Verification items for the finished model (mm, model axes). Face numbers are marked on the shaded views. A direction names the side the tool comes from. Round coordinates to 2 decimals unless told otherwise and drop trailing zeros. Write each loop counter-clockwise with the first axis right and the second up, starting at its lowest first coordinate (ties: lowest second). Pieces come first, ordered by that corner, then holes. Notation, with made-up numbers: M -23.5,9.5 L 4.5,9.5 A11 ccw 4.5,19.5 Z; hole C -4.5,20.5 d7. An arc over 180 degrees is marked long. Answer in a Markdown table with one row per item. Add a question column.
1. Material ranges on probe 1 along Z at (x, y) = (0, 0.55); probe 2 along X at (y, z) = (0.6, 25.5); probe 3 along Y at (x, z) = (0, 26.3), recorded low to high.
2. Sectioned sample at B-B on y = 3.75. Record the cut outline in (x, z).
3. Draft check along Y on the marked faces 1, 2 and 3. Enter one of: pulls with the +Y half, pulls with the -Y half, needs draft (parallel to the pull), parting line crosses it, or undercut.
4. Sectioned sample at A-A on z = 5.5. Record the cut outline in (x, y), plus the area to 3 significant figures.
5. Go/stop test with flat-tipped pins: pin 1 Ø1.2 at (y, z) = (0, 13.5) entering from -X; pin 2 Ø0.5 at (y, z) = (0, 8) entering from +X; pin 3 Ø0.7 at (x, z) = (0, 26) entering from +Y. Record where each tip stops, or that it passes through.
6. Sectioned sample at D-D on z = 25.5. Record the cut outline in (x, y), plus the area to 3 significant figures.
7. Set-up check for the marked faces 4, 5 and 6: record each of +Z, -Z, +X, -X, +Y, -Y from which the full face is reachable in a straight line by a thin tool's end or side.
8. Sectioned sample at C-C on y = 0.5. Record the cut outline in (x, z).
```python
from build123d import *

# Parameters (mm, degrees)
SKETCH1_R                = 0.66
SKETCH1_R_2              = 0.4
BOSS_EXTRUDE1_DEPTH      = 4
BOSS_EXTRUDE1_DEPTH_BACK = 1
BOSS_EXTRUDE2_DEPTH      = 20
SKETCH8_R                = 0.4
BOSS_EXTRUDE3_DEPTH      = 3
BOSS_EXTRUDE3_DEPTH_BACK = 20
FILLET1_R                = 0.5
CUT_EXTRUDE4_START       = -4
CUT_EXTRUDE4_DEPTH       = 4
CUT_EXTRUDE5_START       = -10
CUT_EXTRUDE5_DEPTH       = 4
CUT_EXTRUDE6_START       = -16
CUT_EXTRUDE6_DEPTH       = 4
CUT_EXTRUDE7_DEPTH       = 0.2
CHAMFER1_SIZE            = 0.2
CUT_EXTRUDE9_START       = -22
CUT_EXTRUDE9_DEPTH       = 4
SKETCH17_R               = 0.59
CUT_EXTRUDE11_DEPTH      = 9.61358644


with BuildPart() as part:
    # Sketch1 → Boss-Extrude1 (new body, two sides)
    with BuildSketch(Plane.XY) as boss_extrude1_sk:
        with BuildLine():
            Line((-0.962751438, 1.153198745), (-1.154172794, 0.877795696))
            ThreePointArc((-1.154172794, 0.877795696), (-1.197527345, 0.812911026), (-1.212751438, 0.73637434))
            Line((-1.212751438, 0.73637434), (-1.212751438, -0.81362566))
            Line((-1.212751438, -0.81362566), (0.95, -0.81362566))
            Line((0.95, -0.81362566), (1.2, -0.81362566))
            Line((1.2, -0.81362566), (1.212751438, -0.81362566))
            Line((1.212751438, -0.81362566), (1.212751438, 0.73637434))
            ThreePointArc((1.212751438, 0.73637434), (1.197527345, 0.812911026), (1.154172794, 0.877795696))
            Line((1.154172794, 0.877795696), (0.962751438, 1.153198745))
            Line((0.962751438, 1.153198745), (0.962751438, 2.952748679))
            ThreePointArc((0.962751438, 2.952748679), (1.196528268, 4.111690618), (0.359901995, 4.947067481))
            Line((0.359901995, 4.947067481), (0.359901995, 7.79996078))
            Line((0.359901995, 7.79996078), (-0.340098005, 7.79996078))
            Line((-0.340098005, 7.79996078), (-0.340098005, 4.952843858))
            ThreePointArc((-0.340098005, 4.952843858), (-1.193502974, 4.12155168), (-0.962751438, 2.952748679))
            Line((-0.962751438, 2.952748679), (-0.962751438, 1.153198745))
        make_face()
        with Locations((0, 3.75)):
            Circle(SKETCH1_R, mode=Mode.SUBTRACT)
        with Locations((0, 1.5)):
            Circle(SKETCH1_R_2, mode=Mode.SUBTRACT)
    extrude(amount=BOSS_EXTRUDE1_DEPTH)
    extrude(boss_extrude1_sk.sketch, amount=-BOSS_EXTRUDE1_DEPTH_BACK)

    # Sketch7 → Boss-Extrude2 (add)
    with BuildSketch(Plane.XY.offset(4)):
        with BuildLine():
            Line((-1.154172794, 0.877795696), (1.154172794, 0.877795696))
            ThreePointArc((1.154172794, 0.877795696), (1.197527345, 0.812911026), (1.212751438, 0.73637434))
            Line((1.212751438, 0.73637434), (1.212751438, -0.81362566))
            Line((1.212751438, -0.81362566), (-1.212751438, -0.81362566))
            Line((-1.212751438, -0.81362566), (-1.212751438, 0.73637434))
            ThreePointArc((-1.212751438, 0.73637434), (-1.197527345, 0.812911026), (-1.154172794, 0.877795696))
        make_face()
    extrude(amount=BOSS_EXTRUDE2_DEPTH)

    # Sketch8 → Boss-Extrude3 (add, two sides)
    with BuildSketch(Plane.XY.offset(24)) as boss_extrude3_sk:
        with BuildLine():
            Line((-1.212751438, 0.73637434), (-1.212751438, -0.81362566))
            Line((-1.212751438, -0.81362566), (1.212751438, -0.81362566))
            Line((1.212751438, -0.81362566), (1.212751438, 0.73637434))
            ThreePointArc((1.212751438, 0.73637434), (1.197527345, 0.812911026), (1.154172794, 0.877795696))
            Line((1.154172794, 0.877795696), (0.962751438, 1.153198745))
            Line((0.962751438, 1.153198745), (0.962751438, 2.202748679))
            Line((0.962751438, 2.202748679), (-0.962751438, 2.202748679))
            Line((-0.962751438, 2.202748679), (-0.962751438, 1.153198745))
            Line((-0.962751438, 1.153198745), (-1.154172794, 0.877795696))
            ThreePointArc((-1.154172794, 0.877795696), (-1.197527345, 0.812911026), (-1.212751438, 0.73637434))
        make_face()
        with Locations((0, 1.5)):
            Circle(SKETCH8_R, mode=Mode.SUBTRACT)
    extrude(amount=BOSS_EXTRUDE3_DEPTH)
    extrude(boss_extrude3_sk.sketch, amount=-BOSS_EXTRUDE3_DEPTH_BACK)

    # Fillet1
    fillet1_edges = [part.edges().sort_by_distance(p)[0] for p in [
        (-0.962751438, 2.202748679, 15.5),
        (0.962751438, 2.202748679, 15.5),
    ]]
    fillet(fillet1_edges, radius=FILLET1_R)

    # Sketch10 → Cut-Extrude4 (cut)
    with BuildSketch(Plane.XY.offset(27).offset(CUT_EXTRUDE4_START)):
        Polygon((0, 2.202748679), (0.1, 2.202748679), (0.1, 1.887298335), (-0.1, 1.887298335), (-0.1, 2.202748679), align=None)
    extrude(amount=-CUT_EXTRUDE4_DEPTH, mode=Mode.SUBTRACT)

    # Sketch10_2 → Cut-Extrude5 (cut)
    with BuildSketch(Plane.XY.offset(27).offset(CUT_EXTRUDE5_START)):
        Polygon((0, 2.202748679), (0.1, 2.202748679), (0.1, 1.887298335), (-0.1, 1.887298335), (-0.1, 2.202748679), align=None)
    extrude(amount=-CUT_EXTRUDE5_DEPTH, mode=Mode.SUBTRACT)

    # Sketch10_3 → Cut-Extrude6 (cut)
    with BuildSketch(Plane.XY.offset(27).offset(CUT_EXTRUDE6_START)):
        Polygon((0, 2.202748679), (0.1, 2.202748679), (0.1, 1.887298335), (-0.1, 1.887298335), (-0.1, 2.202748679), align=None)
    extrude(amount=-CUT_EXTRUDE6_DEPTH, mode=Mode.SUBTRACT)

    # Sketch11 → Cut-Extrude7 (cut)
    with BuildSketch(Plane.ZY.offset(-0.1)):
        Polygon((13, 2.202748679), (13, 1.887298335), (12.65, 1.887298335), align=None)
        Polygon((19, 2.202748679), (19, 1.887298335), (18.65, 1.887298335), align=None)
        Polygon((7.000738825, 2.202748679), (7.000738825, 1.887298335), (6.650738825, 1.887298335), align=None)
    extrude(amount=CUT_EXTRUDE7_DEPTH, mode=Mode.SUBTRACT)

    # Chamfer1
    chamfer1_edges = [part.edges().sort_by_distance(p)[0] for p in [
        (-0.4, 1.5, 27),
    ]]
    chamfer(chamfer1_edges, length=CHAMFER1_SIZE)

    # Sketch14 → Cut-Extrude9 (cut)
    with BuildSketch(Plane.XY.offset(27).offset(CUT_EXTRUDE9_START)):
        Polygon((0.2, 1.1), (0.2, -0.81362566), (-0.2, -0.81362566), (-0.2, 1.1), (-0.2, 1.254612966), (0, 1.254612966), (0.2, 1.254612966), align=None)
    extrude(amount=-CUT_EXTRUDE9_DEPTH, mode=Mode.SUBTRACT)

    # Sketch17 → Cut-Extrude11 (cut, through all)
    with BuildSketch(Plane.XZ.offset(0.81362566)):
        with Locations(Location((0, 25.5, 0), (0, 0, 270))):  # turned: the seam where the file's is
            Circle(SKETCH17_R)
    extrude(amount=-CUT_EXTRUDE11_DEPTH, mode=Mode.SUBTRACT)


solid = part.part
```
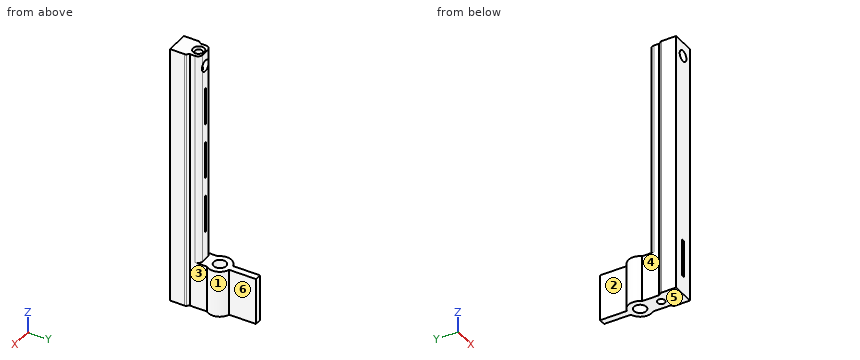
Geometry check:
| question | item | result |
|---|---|---|
| 1 | probe 1 | z = -1 to 1, 5 to 24.91, 26.09 to 27 |
| 1 | probe 2 | x = -1.21 to -0.59, 0.59 to 1.21 |
| 1 | probe 3 | y = -0.81 to 1.1, 1.9 to 2.2 |
| 2 | outline | M -1.25,-1 L -0.66,-1 L -0.66,4 L -1.25,4 Z; M 0.66,-1 L 1.25,-1 L 1.25,4 L 0.66,4 Z |
| 3 | face 1 | undercut |
| 3 | face 2 | needs draft |
| 3 | face 3 | undercut |
| 4 | outline | M -1.21,-0.81 L 1.21,-0.81 L 1.21,0.74 A0.2 ccw 1.15,0.88 L 0.96,1.15 L 0.96,1.7 A0.5 ccw 0.46,2.2 L -0.46,2.2 A0.5 ccw -0.96,1.7 L -0.96,1.15 L -1.15,0.88 A0.2 ccw -1.21,0.74 Z; hole C 0,1.5 d0.8 |
| 4 | area | 6.09 mm2 |
| 5 | pin 1 | stops at x = -1.21 |
| 5 | pin 2 | stops at x = 1.21 |
| 5 | pin 3 | stops at y = 2.2 |
| 6 | outline | M -1.21,-0.81 L -0.59,-0.81 L -0.59,2.19 A0.5 ccw -0.96,1.7 L -0.96,1.15 L -1.15,0.88 A0.2 ccw -1.21,0.74 Z; M 0.59,-0.81 L 1.21,-0.81 L 1.21,0.74 A0.2 ccw 1.15,0.88 L 0.96,1.15 L 0.96,1.7 A0.5 ccw 0.59,2.19 Z |
| 6 | area | 3.04 mm2 |
| 7 | face 4 | +Z, -Z, -X |
| 7 | face 5 | -Z, +X, -X, +Y, -Y |
| 7 | face 6 | +Z, -Z, +X, +Y |
| 8 | outline | M -1.21,-1 L 1.21,-1 L 1.21,27 L -1.21,27 Z; hole C 0,25.5 d1.18; hole M -0.2,1 L 0.2,1 L 0.2,5 L -0.2,5 Z |
